Source: CAD feature listing. Evaluate the final solid. Frame: model axes, mm. Face numbers are marked on the shaded views. A direction names the side the tool comes from. Give positions to 0.01 mm unless a question says otherwise; leave off trailing zeros. Order: outer loops, then holes, each group sorted by start corner. A loop starts at its lowest first (then second) coordinate and runs counter-clockwise, first axis right, second up.
```python
from build123d import *

# Parameters (mm, degrees)
SKETCH1_W           = 100
SKETCH1_H           = 100
BOSS_EXTRUDE1_DEPTH = 100
SKETCH2_R           = 20
CUT_EXTRUDE1_DEPTH  = 4
SKETCH3_W           = 60
SKETCH3_H           = 100
CUT_EXTRUDE2_DEPTH  = 90
SKETCH4_R           = 20
CUT_EXTRUDE3_DEPTH  = 135
FILLET1_R           = 10
FILLET2_R           = 10


with BuildPart() as part:
    # Sketch1 → Boss-Extrude1 (new body)
    with BuildSketch(Plane(origin=(0, 0, 0), x_dir=(1, 0, 0), z_dir=(0, 1, 0))):
        Rectangle(SKETCH1_W, SKETCH1_H)
    extrude(amount=BOSS_EXTRUDE1_DEPTH)

    # Sketch2 → Cut-Extrude1 (cut)
    with BuildSketch(Plane(origin=(0, 100, 0), x_dir=(1, 0, 0), z_dir=(0, 1, 0))):
        with Locations(Location((0, 0, 0), (0, 0, 270))):
            Circle(SKETCH2_R)
    extrude(amount=-CUT_EXTRUDE1_DEPTH, mode=Mode.SUBTRACT)

    # Sketch3 → Cut-Extrude2 (cut)
    with BuildSketch(Plane.XZ):
        Rectangle(SKETCH3_W, SKETCH3_H)
    extrude(amount=-CUT_EXTRUDE2_DEPTH, mode=Mode.SUBTRACT)

    # Sketch4 → Cut-Extrude3 (cut)
    with BuildSketch(Plane.ZY.offset(50)):
        with Locations((0, 40)):
            Circle(SKETCH4_R)
    extrude(amount=-CUT_EXTRUDE3_DEPTH, mode=Mode.SUBTRACT)

    # Fillet1
    fillet1_edges = [part.edges().sort_by_distance(p)[0] for p in [
        (50, 50, 50),
        (-50, 50, 50),
        (-50, 50, -50),
        (50, 50, -50),
    ]]
    fillet(fillet1_edges, radius=FILLET1_R)

    # Fillet2
    fillet2_edges = [part.edges().sort_by_distance(p)[0] for p in [
        (30, 90, 0),
        (-30, 90, 0),
    ]]
    fillet(fillet2_edges, radius=FILLET2_R)


solid = part.part
```
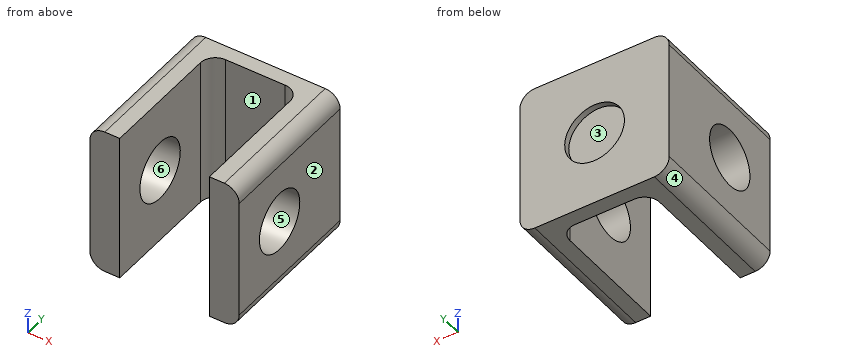
1) Pin query (flat end, axial travel): pin 1 (12 mm diameter, centred on x = 0, z = -21.5, fed in from -Y); pin 2 (1 mm diameter, centred on y = 45.5, z = -17.5, fed in from -X). Return the tip coordinate at first contact, or that it passes through.
Report:
pin 1: stops at y = 90
pin 2: passes through
2) Section query B-B, the plane z = 0. Return the cut outline in (x, y), and give its area (3 significant figures).
Report:
outline: (-50, 0) - (-30, 0) - (-30, 20) - (-50, 20) - close; (-50, 60) - (-30, 60) - (-30, 80) arc R10 cw to (-20, 90) - (20, 90) arc R10 cw to (30, 80) - (30, 60) - (50, 60) - (50, 100) - (20, 100) - (20, 96) - (-20, 96) - (-20, 100) - (-50, 100) - close; (30, 0) - (50, 0) - (50, 20) - (30, 20) - close
area: 2,880 mm2
3) Reachability of the marked faces 1 and 2 from +Z, -Z, +X, -X, +Y, -Y: full face, straight path, thin tool, end or side. Return the list, or none.
Report:
face 1: +Z, -Z, -Y
face 2: +Z, -Z, +X, +Y, -Y
4) Draft query along Y for the marked faces 3, 4, 5 and 6. Return one class per face: +Y half, -Y half, draft (parallel to the pull), parting line (faces both ways), or undercut.
Report:
face 3: +Y half
face 4: draft
face 5: undercut
face 6: undercut
5) Section query D-D, the plane y = 7.5. Return the cut outline in (x, z).
Report:
outline: (-50, -40) arc R10 ccw to (-40, -50) - (-30, -50) - (-30, 50) - (-40, 50) arc R10 ccw to (-50, 40) - close; (30, -50) - (40, -50) arc R10 ccw to (50, -40) - (50, 40) arc R10 ccw to (40, 50) - (30, 50) - close
6) Section query A-A, the plane y = 40. Return the cut outline in (x, z), and give its area (3 significant figures).
Report:
outline: (-50, -40) arc R10 ccw to (-40, -50) - (-30, -50) - (-30, -20) - (-50, -20) - close; (-50, 20) - (-30, 20) - (-30, 50) - (-40, 50) arc R10 ccw to (-50, 40) - close; (30, -50) - (40, -50) arc R10 ccw to (50, -40) - (50, -20) - (30, -20) - close; (30, 20) - (50, 20) - (50, 40) arc R10 ccw to (40, 50) - (30, 50) - close
area: 2,310 mm2
7) Material intervals for L1, parallel to X at y = 26.5, z = 18.5; L2, parallel to Y at x = 36, z = 0; L3, parallel to X at y = 98, z = 0, sorted ascending.
Report:
L1: x = -50 to -30, 30 to 50
L2: y = 0 to 20, 60 to 100
L3: x = -50 to -20, 20 to 50
8) Section query C-C, the plane x = 16. Return the cut outline in (y, z), and give its area (3 significant figures).
Report:
outline: (90, -50) - (100, -50) - (100, -12) - (96, -12) - (96, 12) - (100, 12) - (100, 50) - (90, 50) - close
area: 904 mm2
